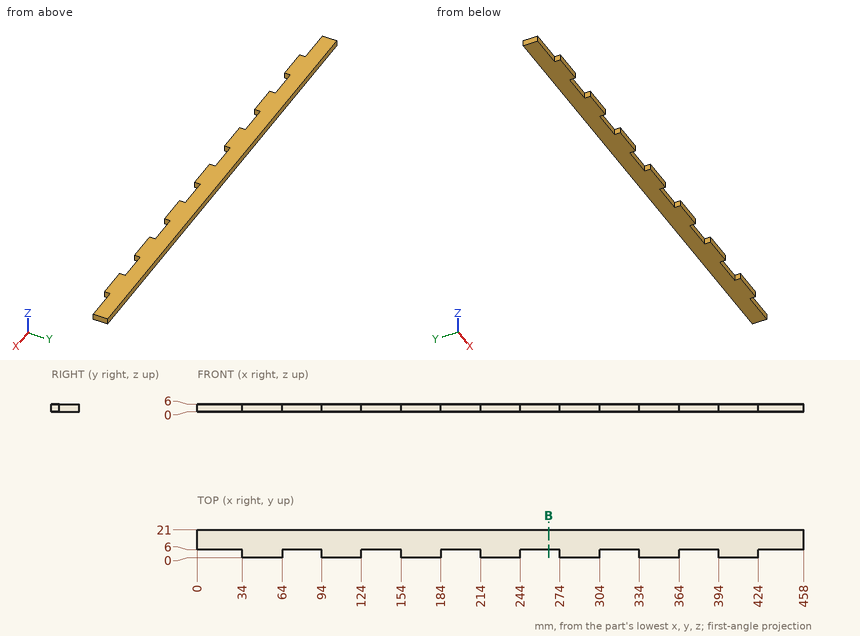
The drawing under review shows one solid part. Ordinate dimensions are in mm from its lowest x, y, z. Give positions to 0.01 mm unless a question says otherwise; leave off trailing zeros. Write each loop counter-clockwise with the first axis right and the second up, starting at its lowest first coordinate (ties: lowest second). Pieces come first, ordered by that corner, then holes. Notation, with made-up numbers: (69, 41.25) -> (100, 41.25) arc R22 ccw to (100, 60.25) -> close; hole circle Ø2 at (-11.5, 21). An arc over 180 degrees is marked (long way). Answer in a Markdown table with one row per item.
(1) Consider section B-B (x = 265.5). State the section outline as (y, z) points, then the cut area to 3 significant figures.
Results:
| item | result |
|---|---|
| outline | (6, 0) -> (21, 0) -> (21, 6) -> (6, 6) -> close |
| area | 90.0 mm2 |
(2) Clearance check with flat-ended pins moving along their axes: pin 1 (1.8 mm diameter, centred on y = 4, z = 3.5, fed in from +X); pin 2 (3 mm diameter, centred on x = 390.5, z = 4.5, fed in from -Y). State where each tip first meets the part, or that it passes through.
Results:
| item | result |
|---|---|
| pin 1 | x = 424 |
| pin 2 | y = 6 |
(3) To check wall thickness, follow probe 1 along Y at (x, z) = (196.5, 4.7). State the ranges of the line that lie inside material, in increasing order.
Results:
| item | result |
|---|---|
| probe 1 | 6 to 21 |
